Autodesk Inventor part; units mm, degrees
ref_plane "YZ Plane" through (0, 0, 0) normal (1, 0, 0) x (0, 1, 0)
ref_plane "XZ Plane" through (0, 0, 0) normal (0, 1, 0) x (-1, 0, 0)
ref_plane "XY Plane" through (0, 0, 0) normal (0, 0, 1) x (1, 0, 0)
sketch "Sketch1" plane through (0, 0, 0) normal (0, 0, 1) x (1, 0, 0)
  circle A0 centre (0, 0) radius 6.1
  line L0 (-12.5, -10) -> (12.5, -10)
  line L1 (12.5, -10) -> (12.5, 10)
  line L2 (12.5, 10) -> (-12.5, 10)
  line L3 (-12.5, 10) -> (-12.5, -10)
  line L4 (-12.5, -10) -> (12.5, 10) construction
  line L5 (12.5, -10) -> (-12.5, 10) construction
  dimension "d0" = 12.2
  dimension "d1" = 25
  dimension "d2" = 20
extrude "Extrusion1" add sketch "Sketch1" along normal blind 20
sketch "Sketch2" plane through (-12.5, 10, 0) normal (0, 1, 0) x (1, 0, 0)
  line L0 (0, 0) -> (0, -20) construction
  line L1 (25, -20) -> (0, -20) construction
  line L2 (0, 0) -> (25, -20) construction
  line L3 (0, -20) -> (25, 0) construction
  circle A0 centre (12.5, -10) radius 1.95
  point P0 (12.5, 0)
  dimension "d5" = 3.9
extrude "Extrusion2" cut sketch "Sketch2" against normal blind 100
sketch "Sketch3" plane through (-12.5, 10, 0) normal (0, 1, 0) x (1, 0, 0)
  circle A0 centre (12.5, -10) radius 1.95
  line L0 (25, 0) -> (0, 0)
  line L1 (0, 0) -> (0, -20)
  line L2 (25, -20) -> (0, -20)
  line L3 (25, 0) -> (25, -20)
  circle A1 centre (12.5, -10) radius 7.5
  point P0 (12.5, 0)
  dimension "d8" = 15
extrude "Extrusion3" add sketch "Sketch3" along normal blind 15 contours A1
sketch "Sketch4" plane through (-12.5, -10, 0) normal (0, -1, 0) x (1, 0, 0)
  line L0 (32.5, 25) -> (-7.5, 25)
  line L1 (-7.5, 25) -> (-7.5, -5)
  line L2 (-7.5, -5) -> (32.5, -5)
  line L3 (32.5, -5) -> (32.5, 25)
  circle A0 centre (12.5, 10) radius 1.95
  line L4 (32.5, 25) -> (-7.5, -5) construction
  line L5 (-7.5, 25) -> (32.5, -5) construction
  point P0 (12.5, 0)
  dimension "d11" = 30
  dimension "d12" = 40
extrude "Extrusion4" add sketch "Sketch4" along normal blind 3
sketch "Sketch6" plane through (20, -10, -5) normal (0, 0, -1) x (-1, 0, 0)
  line L0 (-13.3468, 43.0165) -> (63.7046, 43.0165)
  line L1 (63.7046, 43.0165) -> (63.7046, -16.6019)
  line L2 (63.7046, -16.6019) -> (-13.3468, -16.6019)
  line L3 (-13.3468, -16.6019) -> (-13.3468, 43.0165)
  point P0 (20, 10)
extrude "Extrusion6" cut sketch "Sketch6" against normal blind 10
sketch "Sketch8" plane through (-12.5, 25, 0) normal (0, 1, 0) x (1, 0, 0)
  circle A0 centre (12.5, -10) radius 1.95
  point P0 (12.5, 0)
extrude "Extrusion8" cut sketch "Sketch8" against normal blind 100
sketch "Sketch9" plane through (0, 0, 20) normal (0, 0, 1) x (1, 0, 0)
  line L0 (-2, 5.7628) -> (-2, 3)
  line L1 (-2, 3) -> (2, 3)
  line L2 (2, 3) -> (2, 5.7628)
  circle A0 centre (0, 0) radius 6.1
  line L3 (12.5, -10) -> (12.5, 10)
  line L4 (12.5, 10) -> (-12.5, 10)
  line L5 (-12.5, 10) -> (-12.5, -10)
  line L6 (-12.5, -10) -> (12.5, -10)
  circle A1 centre (0, 0) radius 6.1
  dimension "d28" = 2
  dimension "d29" = 2
  dimension "d30" = 3
extrude "Extrusion9" add sketch "Sketch9" against normal blind 2 contours L0 L1 L2 A0 picked at (0.2259, -0.0207)
sketch "Sketch10" plane through (0, 0, 18) normal (0, 0, -1) x (-1, 0, 0)
  circle A0 centre (0, 0) radius 4.9
  dimension "d33" = 9.8
extrude "Extrusion10" add sketch "Sketch10" along normal blind 15
sketch "Sketch11" plane through (-12.5, 25, 0) normal (0, 1, 0) x (1, 0, 0)
  circle A0 centre (12.5, -10) radius 1.95
  point P0 (12.5, 0)
extrude "Extrusion11" cut sketch "Sketch11" against normal blind 100
properties part number "Primary_hinge_template"
The listing builds one solid part. Answer for the finished solid, in the listing's coordinates (mm). A direction names the side the tool comes from. Round coordinates to 2 decimals unless told otherwise and drop trailing zeros. Write each loop counter-clockwise with the first axis right and the second up, starting at its lowest first coordinate (ties: lowest second). Pieces come first, ordered by that corner, then holes. Notation, with made-up numbers: M -28.75,35 L 15.25,35 A16 cw 15.25,39 Z; hole C 6,-18 d9. An arc over 180 degrees is marked long. Write each question's results on one line, items separated by ' | '. Start each with the question number.
(1) Each of these flat-tipped pins is pushed along its axis until it touches: P1, Ø1, axis at x = 1, y = 4, coming from the +Z side; P2, Ø8, axis at x = 0.5, y = 0, coming from the +Z side; P3, Ø4, axis at x = 13, z = 19.5, coming from the +Y side. Where does it stop, or does it pass through?
(2) For faces 1 (the flat face through (-12.5, 0, 12)), 2 (the cylindrical face through (-4.674, -1.472, 10.605)), 3 (the flat face through (0, 3, 19)), 4 (the flat face through (0, 0, 20)), determine the directions among +Z, -Z, +X, -X, +Y, -Y from which every point of the face is accessible in a straight line to the end or side of a thin tool.
(3) The part is cut by section B-B, the plane x = 0. Give the number of separate pieces and of enclosed holes in the cut face, and give its area (3 significant figures).
(4) Find the intervals of material crossed by line 1 (X direction, y = 0, z = 13.25); line 2 (Z direction, x = 0, y = 2.5); line 3 (X direction, y = -8, z = 10), in increasing order.
(5) Determine the mould class of faces 5 (the flat face through (-1, -5, 18)), 6 (the cylindrical face through (-0.254, 15.524, 8.067)), 7 (the flat face through (3, 10, 17.4)) for opening direction Y: +Y half, -Y half, draft (parallel to the pull), parting line (faces both ways), or undercut.
(6) The part is cut by section D-D, the plane z = 12.75. Write down the section's boundary in (x, y), and give its area (3 significant figures).
(7) The part is cut by section C-C, the plane y = 0. Write down the section's boundary in (x, z), and give its area (3 significant figures).
(8) The part is cut by section A-A, the plane z = 16. Write down the section's boundary in (x, y), and give its area (3 significant figures).
Worked answers:
1) P1: stops at z = 18 | P2: stops at z = 20 | P3: stops at y = 10
2) face 1: +Z, -Z, -X, +Y | face 2: -Z | face 3: +Z | face 4: +Z, +X, -X, +Y
3) separate pieces: 5 | enclosed holes: 0 | area: 391 mm²
4) line 1: x = -12.5 to -6.1, -4.9 to 4.9, 6.1 to 12.5 | line 2: z = 3 to 8.05, 11.95 to 20 | line 3: x = -12.5 to -1.95, 1.95 to 12.5
5) face 5: undercut | face 6: draft | face 7: +Y half
6) outline: M -20,-13 L 20,-13 L 20,-10 L 12.5,-10 L 12.5,10 L 6.98,10 L 6.98,25 L -6.98,25 L -6.98,10 L -12.5,10 L -12.5,-10 L -20,-10 Z; C 0,0 d9.8; hole C 0,0 d12.2 | area: 788 mm²
7) outline: M -12.5,5 L -6.1,5 L -6.1,18 L -4.9,18 L -4.9,3 L 4.9,3 L 4.9,18 L 6.1,18 L 6.1,5 L 12.5,5 L 12.5,20 L -12.5,20 Z; hole C 0,10 d3.9 | area: 351 mm²
8) outline: M -20,-13 L 20,-13 L 20,-10 L 12.5,-10 L 12.5,10 L 4.5,10 L 4.5,25 L -4.5,25 L -4.5,10 L -12.5,10 L -12.5,-10 L -20,-10 Z; C 0,0 d9.8; hole C 0,0 d12.2 | area: 714 mm²
